Input: dimensioned drawing with shaded views. Units: mm. Origin: part minimum x, y, z. Round coordinates to 2 decimals unless told otherwise and drop trailing zeros. Loops run counter-clockwise (first coordinate to the right, second up) from the corner with the lowest first, then second, coordinate; pieces in that order, holes last.
Item 1: Section query A-A on x = 35.4. Return loops of the section in (y, z), then the cut area to 3 significant figures.
Item 2: Pull-direction query (X, two-part tool) for the marked faces 1, 2 and 3; classes: released by +X, released by -X, zero draft, split by the parting line, or undercut.
Item 3: Section query D-D on z = 1.75. Return loops of the section in (x, y), then the cut area to 3 significant figures.
Item 4: First-contact query: P1, Ø3, axis at y = 46.5, z = 3, coming from the +X side; P2, Ø1, axis at y = 33, z = 2.5, coming from the +X side; P3, Ø2, axis at x = 31, z = 2, coming from the +Y side; P4, Ø1.8, axis at x = 35.4, y = 65.8, coming from the +Z side. Flat tips, straight axial feed; report the tip coordinate or a pass-through.
Item 5: Section query C-C on x = 65.8. Return loops of the section in (y, z).
Item 6: Ray query, L1, parallel to Y at x = 35.4, z = 2.75; L2, parallel to X at y = 36.5, z = 3.75. Return the intervals inside material, ascending.
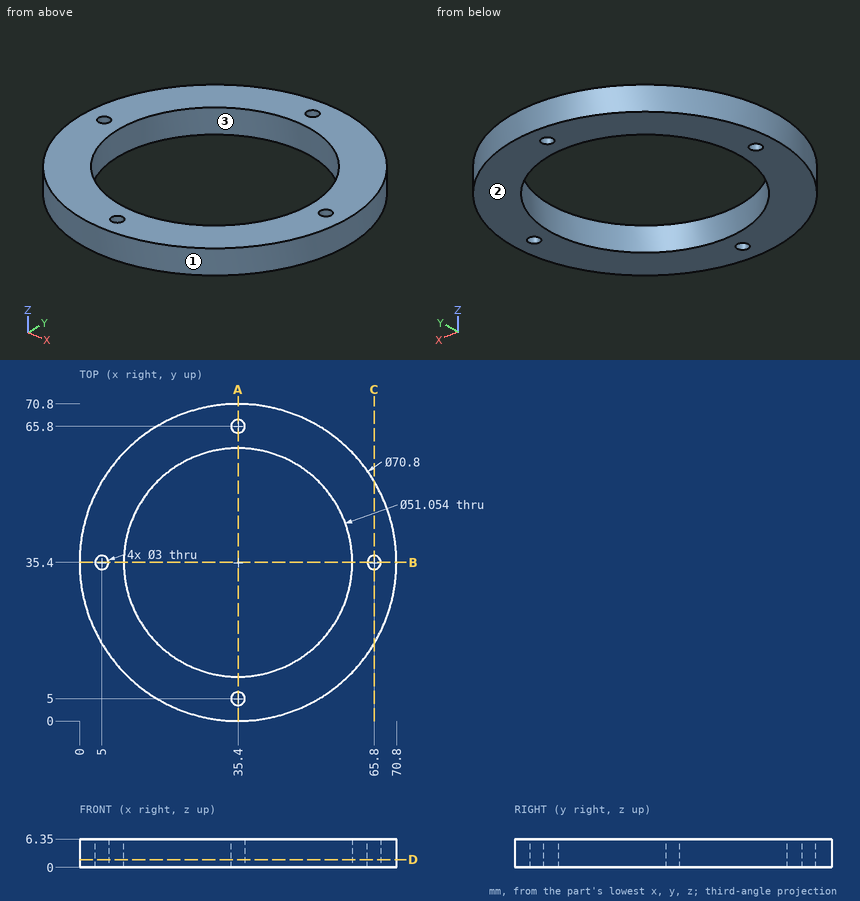
Data:
1. outline: (0, 0) - (3.5, 0) - (3.5, 6.35) - (0, 6.35) - close; (6.5, 0) - (9.87, 0) - (9.87, 6.35) - (6.5, 6.35) - close; (60.93, 0) - (64.3, 0) - (64.3, 6.35) - (60.93, 6.35) - close; (67.3, 0) - (70.8, 0) - (70.8, 6.35) - (67.3, 6.35) - close
1. area: 87.3 mm2
2. face 1: split by the parting line
2. face 2: zero draft
2. face 3: undercut
3. outline: circle Ø70.8 at (35.4, 35.4); hole circle Ø3 at (5, 35.4); hole circle Ø51.05 at (35.4, 35.4); hole circle Ø3 at (35.4, 5); hole circle Ø3 at (35.4, 65.8); hole circle Ø3 at (65.8, 35.4)
3. area: 1,860 mm2
4. P1: stops at x = 69.47
4. P2: stops at x = 70.75
4. P3: stops at y = 70.64
4. P4: passes through
5. outline: (17.26, 0) - (33.9, 0) - (33.9, 6.35) - (17.26, 6.35) - close; (36.9, 0) - (53.54, 0) - (53.54, 6.35) - (36.9, 6.35) - close
6. L1: y = 0 to 3.5, 6.5 to 9.87, 60.93 to 64.3, 67.3 to 70.8
6. L2: x = 0.02 to 3.98, 6.02 to 9.9, 60.9 to 64.78, 66.82 to 70.78
